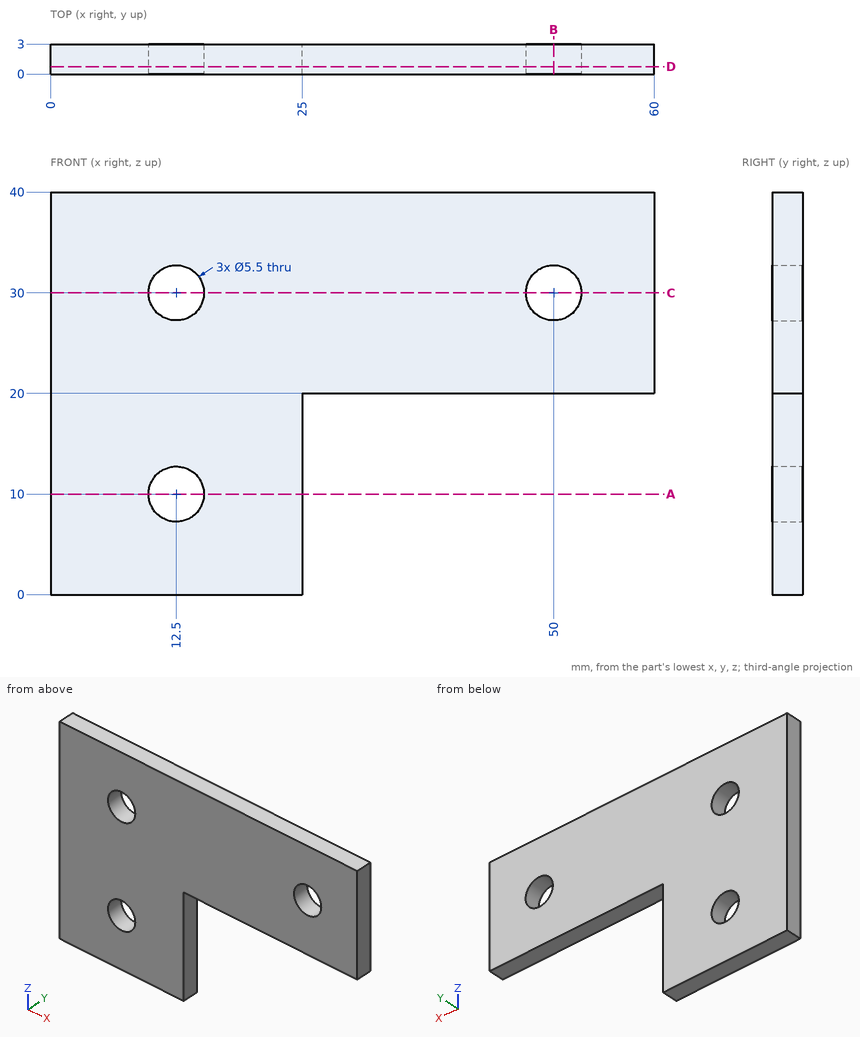
Design review of the part shown in the three views and the two pictorial views. Dimensions are in mm from the part's minimum x, y and z. Give positions to 0.01 mm unless a question says otherwise; leave off trailing zeros. Write each loop counter-clockwise with the first axis right and the second up, starting at its lowest first coordinate (ties: lowest second). Pieces come first, ordered by that corner, then holes.
(1) Add section C-C (z = 30). Give the boundary of the cut face in (x, y).
Checked values:
outline: (0, 0) - (9.75, 0) - (9.75, 3) - (0, 3) - close; (15.25, 0) - (47.25, 0) - (47.25, 3) - (15.25, 3) - close; (52.75, 0) - (60, 0) - (60, 3) - (52.75, 3) - close
(2) Wall thickness on line 1 along X through (y, z) = (1.25, 30); line 2 along Z through (x, y) = (12.5, 1.15); line 3 along X through (y, z) = (0.35, 10): over which ranges is each line inside the solid? List them lowest first.
Checked values:
line 1: x = 0 to 9.75, 15.25 to 47.25, 52.75 to 60
line 2: z = 0 to 7.25, 12.75 to 27.25, 32.75 to 40
line 3: x = 0 to 9.75, 15.25 to 25
(3) Add section B-B (x = 50). Give the boundary of the cut face in (y, z), and give its area (3 significant figures).
Checked values:
outline: (0, 20) - (3, 20) - (3, 27.25) - (0, 27.25) - close; (0, 32.75) - (3, 32.75) - (3, 40) - (0, 40) - close
area: 43.5 mm2
(4) Clearance check with flat-ended pins moving along their axes: pin 1 Ø7 at (x, z) = (50, 30) entering from -Y; pin 2 Ø0.9 at (x, y) = (45.5, 2) entering from -Z. State where each tip first meets the part, or that it passes through.
Checked values:
pin 1: stops at y = 0
pin 2: stops at z = 20
(5) Add section D-D (y = 0.75). Give the boundary of the cut face in (x, z).
Checked values:
outline: (0, 0) - (25, 0) - (25, 20) - (60, 20) - (60, 40) - (0, 40) - close; hole circle Ø5.5 at (12.5, 10); hole circle Ø5.5 at (12.5, 30); hole circle Ø5.5 at (50, 30)
(6) Add section A-A (z = 10). Give the boundary of the cut face in (x, y), and give its area (3 significant figures).
Checked values:
outline: (0, 0) - (9.75, 0) - (9.75, 3) - (0, 3) - close; (15.25, 0) - (25, 0) - (25, 3) - (15.25, 3) - close
area: 58.5 mm2
